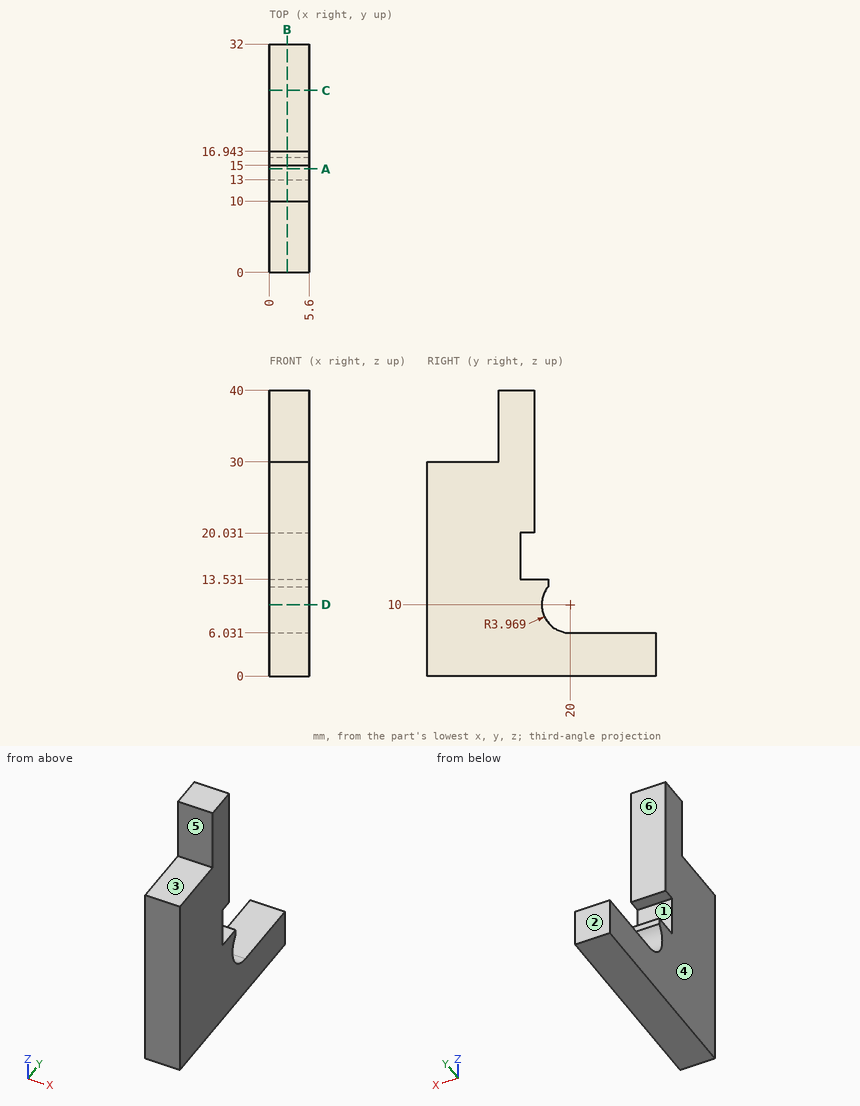
Print and shaded views of the part. All mm, measured from the part's lowest x, y and z. A direction names the side the tool comes from. Coordinates: 2 decimals unless noted, no trailing zeros. Loops run counter-clockwise (first coordinate to the right, second up) from the corner with the lowest first, then second, coordinate; pieces in that order, holes last. Notation, with made-up numbers: (-13, 76.25) -> (8, 76.25) arc R10 cw to (8, 93.25) -> close; hole circle Ø1 at (46, -31). An arc over 180 degrees is marked (long way). Use a Markdown table: item, result. Add a question column.
Item 1: Band-saw the part on B-B on x = 2.5. Write the cut outline in (y, z), plus the area to 3 significant figures.
Item 2: Band-saw the part on A-A on y = 14.5. Write the cut outline in (x, z), plus the area to 3 significant figures.
Item 3: Probe probe 1 along Z at (x, y) = (0.35, 23); probe 2 along Z at (x, y) = (2, 16); probe 3 along Y at (x, z) = (4.5, 18.5). List the from-to ranges inside material, lowest first.
Item 4: Pull direction Z, two halves, no side cores. Call the marked faces 1, 2 and 3: +Z half, -Z half, draft (parallel to the pull), parting line (faces both ways), or undercut.
Item 5: Flat gauge pins, fed straight in: P1, Ø1.7, axis at x = 2, z = 30.5, coming from the +Y side; P2, Ø0.5, axis at x = 2.5, z = 13, coming from the +Y side; P3, Ø3, axis at x = 2.5, z = 36.5, coming from the -Y side. Where does each tip first touch, or does it go through?
Item 6: Which spindle directions (+Z, -Z, +X, -X, +Y, -Y) get a long thin tool onto all of the face, cutting with end or side? Do the marked faces 4, 5 and 6. Say none if no direction does.
Item 7: Band-saw the part on D-D on z = 10. Write the cut outline in (x, y).
Item 8: Band-saw the part on C-C on y = 25.5. Write the cut outline in (x, z).
Geometry says:
| question | item | result |
|---|---|---|
| 1 | outline | (0, 0) -> (32, 0) -> (32, 6.03) -> (20, 6.03) arc R3.97 cw to (16.94, 12.53) -> (16.94, 13.53) -> (13, 13.53) -> (13, 20.03) -> (15, 20.03) -> (15, 40) -> (10, 40) -> (10, 30) -> (0, 30) -> close |
| 1 | area | 602 mm² |
| 2 | outline | (0, 0) -> (5.6, 0) -> (5.6, 13.53) -> (0, 13.53) -> close; (0, 20.03) -> (5.6, 20.03) -> (5.6, 40) -> (0, 40) -> close |
| 2 | area | 188 mm² |
| 3 | probe 1 | 0 to 6.03 |
| 3 | probe 2 | 0 to 13.53 |
| 3 | probe 3 | 0 to 13 |
| 4 | face 1 | undercut |
| 4 | face 2 | draft |
| 4 | face 3 | +Z half |
| 5 | P1 | y = 15 |
| 5 | P2 | y = 16.94 |
| 5 | P3 | y = 10 |
| 6 | face 4 | +Z, -Z, -X, +Y, -Y |
| 6 | face 5 | +Z, +X, -X, -Y |
| 6 | face 6 | +Z, +X, -X, +Y |
| 7 | outline | (0, 0) -> (5.6, 0) -> (5.6, 16.03) -> (0, 16.03) -> close |
| 8 | outline | (0, 0) -> (5.6, 0) -> (5.6, 6.03) -> (0, 6.03) -> close |
